Check sheet for the modelled part. Datum: model origin and axes. Units: mm. A direction names the side the tool comes from. Give positions to 0.01 mm unless a question says otherwise; leave off trailing zeros. Write each loop counter-clockwise with the first axis right and the second up, starting at its lowest first coordinate (ties: lowest second). Pieces come first, ordered by that corner, then holes.
from build123d import *

# Parameters (mm, degrees)
SKETCH1_R             = 1.45
BOSS_EXTRUDE1_DEPTH   = 2.2
BOSS_EXTRUDE1_2_DEPTH = 2.2
SKETCH8_W             = 6
SKETCH8_H             = 5.9
BOSS_EXTRUDE6_DEPTH   = 42
BOSS_EXTRUDE7_DEPTH   = 5
SKETCH10_W            = 31
SKETCH10_H            = 3
BOSS_EXTRUDE8_DEPTH   = 53.85
SKETCH11_W            = 31
SKETCH11_H            = 35.214875224
SKETCH11_R            = 0.925
BOSS_EXTRUDE9_DEPTH   = 4
CHAMFER6_SIZE         = 19.1
CHAMFER7_SIZE         = 12
CHAMFER8_SIZE         = 2
CUT_EXTRUDE2_START    = 2
CUT_EXTRUDE2_DEPTH    = 27
CHAMFER10_SIZE        = 0.8
SKETCH14_W            = 7.5
SKETCH14_H            = 5.9
CUT_EXTRUDE3_DEPTH    = 112.547893301
CHAMFER11_SIZE        = 5
CHAMFER11_SIZE2       = 28.356409098
SKETCH15_W            = 2
SKETCH15_H            = 27.75
BOSS_EXTRUDE10_DEPTH  = 2.5
BOSS_EXTRUDE11_DEPTH  = 6.5
CHAMFER12_SIZE        = 1
CHAMFER13_SIZE        = 5.5
CHAMFER14_SIZE        = 1.464101615
CHAMFER14_SIZE_2      = 2
CHAMFER15_SIZE        = 0.4


# Some blends are built 0.0001 mm under size
with BuildPart() as part:
    # Sketch1 → Boss-Extrude1 (new body)
    with BuildSketch(Plane.XY):
        Polygon((0, 0), (0, 5.9), (12.25, 5.9), (12.25, 0), (2.5, 0), align=None)
        with Locations((9.4, 2.95)):
            Circle(SKETCH1_R, mode=Mode.SUBTRACT)
    extrude(amount=BOSS_EXTRUDE1_DEPTH)



with BuildPart() as body_2:
    # Sketch1 → Boss-Extrude1 2 (new body)
    with BuildSketch(Plane.XY):
        Polygon((31, 0), (31, 5.9), (18.75, 5.9), (18.75, 0), (28.5, 0), align=None)
        with Locations((21.6, 2.95)):
            Circle(SKETCH1_R, mode=Mode.SUBTRACT)
    extrude(amount=BOSS_EXTRUDE1_2_DEPTH)


with BuildPart() as part_1:
    add(part.part)

    add(body_2.part)  # Boss-Extrude6 merges body 2
    # Sketch8 → Boss-Extrude6 (add)
    with BuildSketch(Plane.XY.offset(2.2)):
        with Locations((3, 2.95)):
            Rectangle(SKETCH8_W, SKETCH8_H)
        with Locations((28, 2.95)):
            Rectangle(SKETCH8_W, SKETCH8_H)
    extrude(amount=BOSS_EXTRUDE6_DEPTH)

    # Sketch9 → Boss-Extrude7 (add)
    with BuildSketch(Plane.XY.offset(44.2)):
        Polygon((0, 5.9), (0, -22.1), (31, -22.1), (31, 5.9), (25, 5.9), (25, -19.1), (6, -19.1), (6, 5.9), align=None)
    extrude(amount=BOSS_EXTRUDE7_DEPTH)

    # Sketch10 → Boss-Extrude8 (add)
    with BuildSketch(Plane.XY.offset(49.2)):
        with Locations((15.5, -20.6)):
            Rectangle(SKETCH10_W, SKETCH10_H)
    extrude(amount=BOSS_EXTRUDE8_DEPTH)

    # Sketch11 → Boss-Extrude9 (add)
    with BuildSketch(Plane.XY.offset(103.05)):
        with Locations((15.5, -4.492562388)):
            Rectangle(SKETCH11_W, SKETCH11_H)
        with Locations((15.5, -3.45)):
            Circle(SKETCH11_R, mode=Mode.SUBTRACT)
        with Locations(Location((15.5, 9.35, 0), (0, 0, 180))):
            Circle(SKETCH11_R, mode=Mode.SUBTRACT)
    extrude(amount=BOSS_EXTRUDE9_DEPTH)

    # Chamfer6
    chamfer6_edges = [part_1.edges().sort_by_distance(p)[0] for p in [
        (3, -19.1, 49.2),
        (28, -19.1, 49.2),
    ]]
    chamfer(chamfer6_edges, length=CHAMFER6_SIZE)

    # Chamfer7
    chamfer7_edges = [part_1.edges().sort_by_distance(p)[0] for p in [
        (15.5, -19.1, 103.05),
    ]]
    chamfer(chamfer7_edges, length=CHAMFER7_SIZE)

    # Chamfer8
    chamfer8_edges = [part_1.edges().sort_by_distance(p)[0] for p in [
        (0, -4.492562388, 107.05),
        (31, -4.492562388, 107.05),
        (15.5, 13.114875224, 107.05),
        (0, 13.114875224, 105.05),
        (31, 13.114875224, 105.05),
        (31, 5.9, 24.6),
        (3, 5.9, 49.2),
        (28, 5.9, 49.2),
        (0, 5.9, 24.6),
    ]]
    chamfer(chamfer8_edges, length=CHAMFER8_SIZE)

    # Sketch13 → Cut-Extrude2 (cut)
    with BuildSketch(Plane(origin=(0, 0, 0), x_dir=(0, 0, -1), z_dir=(1, 0, 0)).offset(CUT_EXTRUDE2_START)):
        Polygon((-103.05, -7.1), (-91.05, -19.1), (-103.05, -19.1), align=None)
    extrude(amount=CUT_EXTRUDE2_DEPTH, mode=Mode.SUBTRACT)

    # Chamfer10
    chamfer10_edges = [part_1.edges().sort_by_distance(p)[0] for p in [
        (6, 2.95, 2.2),
        (25, 2.95, 2.2),
    ]]
    chamfer(chamfer10_edges, length=CHAMFER10_SIZE)

    # Sketch14 → Cut-Extrude3 (cut, through all)
    with BuildSketch(Plane.XY.offset(2.2)):
        with Locations((15.5, 2.95)):
            Rectangle(SKETCH14_W, SKETCH14_H)
    extrude(amount=-CUT_EXTRUDE3_DEPTH, mode=Mode.SUBTRACT)

    # Chamfer11
    chamfer11_edges = [part_1.edges().sort_by_distance(p)[0] for p in [
        (3, 0, 44.2),
        (28, 0, 44.2),
    ]]
    chamfer11_side = [part_1.faces().sort_by_distance(p)[0] for p in [
        (3, -0.380711177, 44.2),
    ]]
    chamfer(chamfer11_edges, length=CHAMFER11_SIZE, length2=CHAMFER11_SIZE2, reference=chamfer11_side[0])

    # Sketch15 → Boss-Extrude10 (add)
    with BuildSketch(Plane(origin=(0, -19.1, 0), x_dir=(1, 0, 0), z_dir=(0, 1, 0))):
        with Locations((1, -79.675)):
            Rectangle(SKETCH15_W, SKETCH15_H)
        with Locations((30, -79.675)):
            Rectangle(SKETCH15_W, SKETCH15_H)
    extrude(amount=BOSS_EXTRUDE10_DEPTH)

    # Sketch16 → Boss-Extrude11 (add)
    with BuildSketch(Plane.XZ.offset(22.1)):
        Polygon((2, 107.05), (2, 44.2), (0, 44.2), (0, 105.05), align=None)
        Polygon((29, 107.05), (29, 44.2), (31, 44.2), (31, 105.05), align=None)
    extrude(amount=BOSS_EXTRUDE11_DEPTH)

    # Chamfer12
    chamfer12_edges = [part_1.edges().sort_by_distance(p)[0] for p in [
        (29, -28.6, 75.625),
        (2, -28.6, 75.625),
    ]]
    chamfer(chamfer12_edges, length=CHAMFER12_SIZE)

    # Chamfer13
    chamfer13_edges = [part_1.edges().sort_by_distance(p)[0] for p in [
        (29, -22.1, 75.625),
        (2, -22.1, 75.625),
    ]]
    chamfer(chamfer13_edges, length=CHAMFER13_SIZE - 0.0001)  # a hair under: the kernel refuses the full size

    # Chamfer14
    # the kernel refuses this chamfer: 2, 1.464101615 mm, written as the material it takes off along each edge
    with BuildSketch(Plane(origin=(32.969523731, -31.569523731, 103.080476269), x_dir=(0.44444688362373996, 0.8153930851078324, -0.37094620148409235), z_dir=(-0.5773502691896258, 0.5773502691896258, 0.5773502691896258)), Plane(origin=(4.969523731, -24.630476269, 110.019523731), x_dir=(-0.4444468836237367, 0.8153930851078325, -0.37094620148409596), z_dir=(-0.5773502691896257, -0.5773502691896258, -0.5773502691896257))) as chamfer14_piece_1:
        Polygon((CHAMFER14_SIZE * 0.998648499248, CHAMFER14_SIZE * 0.0519728307677), (CHAMFER14_SIZE_2 * 0.45431445783, CHAMFER14_SIZE_2 * 0.8908413851), (0, 0), align=None)
    extrude(amount=12.018782759, mode=Mode.SUBTRACT)
    with BuildSketch(Plane(origin=(19.86319104, -18.46309104, 107.05), x_dir=(0.7068394360706733, 0.7068394360706733, 0.027495876610589075), z_dir=(0.7071067811865476, -0.7071067811865476, 0))) as chamfer14_piece_2_section:
        Polygon((CHAMFER14_SIZE_2 * 0.999621916911, -CHAMFER14_SIZE_2 * 0.0274958766106), (-CHAMFER14_SIZE_2 * 0.0274958766106, -CHAMFER14_SIZE_2 * 0.999621916911), (0, 0), align=None)
    chamfer14_piece_2 = extrude(amount=18.064765124, mode=Mode.PRIVATE)
    chamfer14_piece_2 = split(chamfer14_piece_2, bisect_by=Plane(origin=(26.660831265, -22.1, 106.348363543), z_dir=(0, -1, 0)), keep=Keep.TOP, mode=Mode.PRIVATE)
    add(chamfer14_piece_2, mode=Mode.SUBTRACT)
    with BuildSketch(Plane(origin=(2.356534024, -22.1, 107.05), x_dir=(0, 0.9996219169112968, 0.0274958766105891), z_dir=(1, 0, 0))) as chamfer14_piece_3_section:
        Polygon((CHAMFER14_SIZE_2 * 0.999621916911, -CHAMFER14_SIZE_2 * 0.0274958766106), (-CHAMFER14_SIZE_2 * 0.0274958766106, -CHAMFER14_SIZE_2 * 0.999621916911), (0, 0), align=None)
    chamfer14_piece_3 = extrude(amount=26.286931952, mode=Mode.PRIVATE)
    chamfer14_piece_3 = split(chamfer14_piece_3, bisect_by=Plane(origin=(19.18755831, -17.78745831, 106.371913367), z_dir=(-0.7071067811865476, -0.7071067811865476, 0)), keep=Keep.TOP, mode=Mode.PRIVATE)
    chamfer14_piece_3 = split(chamfer14_piece_3, bisect_by=Plane(origin=(11.81244169, -17.78745831, 106.371913367), z_dir=(0.7071067811865476, -0.7071067811865476, 0)), keep=Keep.TOP, mode=Mode.PRIVATE)
    add(chamfer14_piece_3, mode=Mode.SUBTRACT)
    with BuildSketch(Plane(origin=(-1.63690896, -31.23680896, 107.05), x_dir=(-0.7068394360706735, 0.7068394360706735, 0.02749587661058907), z_dir=(0.7071067811865476, 0.7071067811865476, 0))) as chamfer14_piece_4_section:
        Polygon((CHAMFER14_SIZE_2 * 0.999621916911, -CHAMFER14_SIZE_2 * 0.0274958766106), (-CHAMFER14_SIZE_2 * 0.0274958766106, -CHAMFER14_SIZE_2 * 0.999621916911), (0, 0), align=None)
    chamfer14_piece_4 = extrude(amount=18.064765124, mode=Mode.PRIVATE)
    chamfer14_piece_4 = split(chamfer14_piece_4, bisect_by=Plane(origin=(-0.06712973, -22.1, 106.41381375), z_dir=(0, -1, 0)), keep=Keep.TOP, mode=Mode.PRIVATE)
    add(chamfer14_piece_4, mode=Mode.SUBTRACT)
    with BuildSketch(Plane(origin=(6.143365976, -28.6, 44.2), x_dir=(0, 0.9996219169112968, -0.027495876610585647), z_dir=(-1, 0, 0))) as chamfer14_piece_5:
        Polygon((CHAMFER14_SIZE_2 * 0.999621916911, -CHAMFER14_SIZE_2 * 0.0274958766106), (-CHAMFER14_SIZE_2 * 0.0274958766106, -CHAMFER14_SIZE_2 * 0.999621916911), (0, 0), align=None)
    extrude(amount=11.286731952, mode=Mode.SUBTRACT)
    with BuildSketch(Plane(origin=(24.856634024, -28.6, 44.2), x_dir=(0, 0.9996219169112968, -0.027495876610585647), z_dir=(1, 0, 0))) as chamfer14_piece_6:
        Polygon((CHAMFER14_SIZE_2 * 0.999621916911, CHAMFER14_SIZE_2 * 0.0274958766106), (-CHAMFER14_SIZE_2 * 0.0274958766106, CHAMFER14_SIZE_2 * 0.999621916911), (0, 0), align=None)
    extrude(amount=11.286731952, mode=Mode.SUBTRACT)
    with BuildSketch(Plane(origin=(2.356534024, -22.1, 107.05), x_dir=(0, 0.9996219169112968, 0.0274958766105891), z_dir=(1, 0, 0))) as chamfer14_piece_7a_section:
        Polygon((CHAMFER14_SIZE_2 * 0.999621916911, -CHAMFER14_SIZE_2 * 0.0274958766106), (-CHAMFER14_SIZE_2 * 0.0274958766106, -CHAMFER14_SIZE_2 * 0.999621916911), (0, 0), align=None)
    chamfer14_piece_7a = extrude(amount=26.286931952, mode=Mode.PRIVATE)
    chamfer14_piece_7a = split(chamfer14_piece_7a, bisect_by=Plane(origin=(24.258421627, -22.858321627, 106.41381375), z_dir=(0.7071067811865476, 0.7071067811865476, 0)), keep=Keep.TOP, mode=Mode.PRIVATE)
    with BuildSketch(Plane(origin=(19.86319104, -18.46309104, 107.05), x_dir=(0.7068394360706733, 0.7068394360706733, 0.027495876610589075), z_dir=(0.7071067811865476, -0.7071067811865476, 0))) as chamfer14_piece_7b_section:
        Polygon((CHAMFER14_SIZE_2 * 0.999621916911, -CHAMFER14_SIZE_2 * 0.0274958766106), (-CHAMFER14_SIZE_2 * 0.0274958766106, -CHAMFER14_SIZE_2 * 0.999621916911), (0, 0), align=None)
    chamfer14_piece_7b = extrude(amount=18.064765124, mode=Mode.PRIVATE)
    chamfer14_piece_7b = split(chamfer14_piece_7b, bisect_by=Plane(origin=(22.427671271, -22.1, 106.41381375), z_dir=(0, 1, 0)), keep=Keep.TOP, mode=Mode.PRIVATE)
    chamfer14_piece_7 = chamfer14_piece_7a & chamfer14_piece_7b
    add(chamfer14_piece_7, mode=Mode.SUBTRACT)
    with BuildSketch(Plane(origin=(2.356534024, -22.1, 107.05), x_dir=(0, 0.9996219169112968, 0.0274958766105891), z_dir=(1, 0, 0))) as chamfer14_piece_8a_section:
        Polygon((CHAMFER14_SIZE_2 * 0.999621916911, -CHAMFER14_SIZE_2 * 0.0274958766106), (-CHAMFER14_SIZE_2 * 0.0274958766106, -CHAMFER14_SIZE_2 * 0.999621916911), (0, 0), align=None)
    chamfer14_piece_8a = extrude(amount=26.286931952, mode=Mode.PRIVATE)
    chamfer14_piece_8a = split(chamfer14_piece_8a, bisect_by=Plane(origin=(6.741578373, -22.858321627, 106.41381375), z_dir=(-0.7071067811865476, 0.7071067811865476, 0)), keep=Keep.TOP, mode=Mode.PRIVATE)
    with BuildSketch(Plane(origin=(-1.63690896, -31.23680896, 107.05), x_dir=(-0.7068394360706735, 0.7068394360706735, 0.02749587661058907), z_dir=(0.7071067811865476, 0.7071067811865476, 0))) as chamfer14_piece_8b_section:
        Polygon((CHAMFER14_SIZE_2 * 0.999621916911, -CHAMFER14_SIZE_2 * 0.0274958766106), (-CHAMFER14_SIZE_2 * 0.0274958766106, -CHAMFER14_SIZE_2 * 0.999621916911), (0, 0), align=None)
    chamfer14_piece_8b = extrude(amount=18.064765124, mode=Mode.PRIVATE)
    chamfer14_piece_8b = split(chamfer14_piece_8b, bisect_by=Plane(origin=(8.572328729, -22.1, 106.41381375), z_dir=(0, 1, 0)), keep=Keep.TOP, mode=Mode.PRIVATE)
    chamfer14_piece_8 = chamfer14_piece_8a & chamfer14_piece_8b
    add(chamfer14_piece_8, mode=Mode.SUBTRACT)

    # Chamfer15
    chamfer15_edges = [part_1.edges().sort_by_distance(p)[0] for p in [
        (0, -28.6, 75.083267831),
        (31, -28.6, 75.083267831),
    ]]
    chamfer(chamfer15_edges, length=CHAMFER15_SIZE)


solid = part_1.part
1) Sectioned sample at A-A on x = 21.6. Record the boundary of the cut face in (y, z), then the cut area to 3 significant figures.
2) Gauge pin test, flat ends, axial feed: pin 1 (10.5 mm diameter, centred on x = 22.5, z = 27, fed in from +Y); pin 2 (6 mm diameter, centred on x = 26.5, z = 8.5, fed in from -Y); pin 3 (5 mm diameter, centred on x = 11.5, z = 62, fed in from -Y); pin 4 (1 mm diameter, centred on x = 7, z = 21, fed in from +Y). Record the tip position at first contact, or that the pin passes through.
3) Sectioned sample at D-D on x = 5. Record the boundary of the cut face in (y, z), then the cut area to 3 significant figures.
4) Access from +Z, -Z, +X, -X, +Y, -Y to the whole of each face (thin tool, end or side, straight path). Record for faces 4 (the flat face through (1.073, -27.618, 104.916)), 5 (the flat face through (28, 0, 8)), 6 (the flat face through (3, 2, 49.2)), 7 (the flat face through (23.3, 3, 2.2)), 8 (the flat face through (15, -19.1, 73)).
5) Draft check along X on faces 1 (the flat face through (0.99, -8.07, 106.04)), 2 (the flat face through (1, -16.6, 79)), 3 (the flat face through (19.25, 3, 1)). Enter one of: +X half, -X half, draft (parallel to the pull), parting line (faces both ways), or undercut.
6) Scan lines: L1, parallel to X at y = -18, z = 74.5; L2, parallel to Z at x = 23.5, y = 5; L3, parallel to Z at x = 10, y = -2.5. Record each from-to range of solid material in increasing order.
7) Sectioned sample at B-B on y = -10. Record the boundary of the cut face in (x, z), then the cut area to 3 significant figures.
Answers below:
1. outline: (-22.1, 44.2) - (-19.1, 44.2) - (-19.1, 103.05) - (13.11, 103.05) - (13.11, 105.05) - (11.11, 107.05) - (-20.1, 107.05) - (-22.1, 105.05) - close; (0, 0) - (1.5, 0) - (1.5, 2.2) - (0, 2.2) - close; (4.4, 0) - (5.9, 0) - (5.9, 2.2) - (4.4, 2.2) - close
1. area: 320 mm2
2. pin 1: stops at y = 5.9
2. pin 2: stops at y = 0
2. pin 3: stops at y = -22.1
2. pin 4: passes through
3. outline: (-24.6, 44.2) - (-5, 44.2) - (0, 15.84) - (0, 0) - (5.9, 0) - (5.9, 47.2) - (3.9, 49.2) - (0, 49.2) - (-19.1, 68.3) - (-19.1, 103.05) - (13.11, 103.05) - (13.11, 105.05) - (11.11, 107.05) - (-21.77, 107.05) - (-24.6, 105.05) - close
3. area: 1,110 mm2
4. face 4: +Z, -Y
4. face 5: -Z, +X, -X, -Y
4. face 6: +X, -X, +Y
4. face 7: +Y, -Y
4. face 8: +Y
5. face 1: -X half
5. face 2: draft
5. face 3: undercut
6. L1: x = 0 to 2, 29 to 31
6. L2: z = 0 to 2.2, 103.05 to 107.05
6. L3: z = 103.05 to 107.05
7. outline: (0, 44.2) - (6, 44.2) - (6, 59.2) - (0, 59.2) - close; (0, 100.15) - (2, 100.15) - (2, 103.05) - (29, 103.05) - (29, 100.15) - (31, 100.15) - (31, 105.05) - (29, 107.05) - (2, 107.05) - (0, 105.05) - close; (25, 44.2) - (31, 44.2) - (31, 59.2) - (25, 59.2) - close
7. area: 312 mm2
